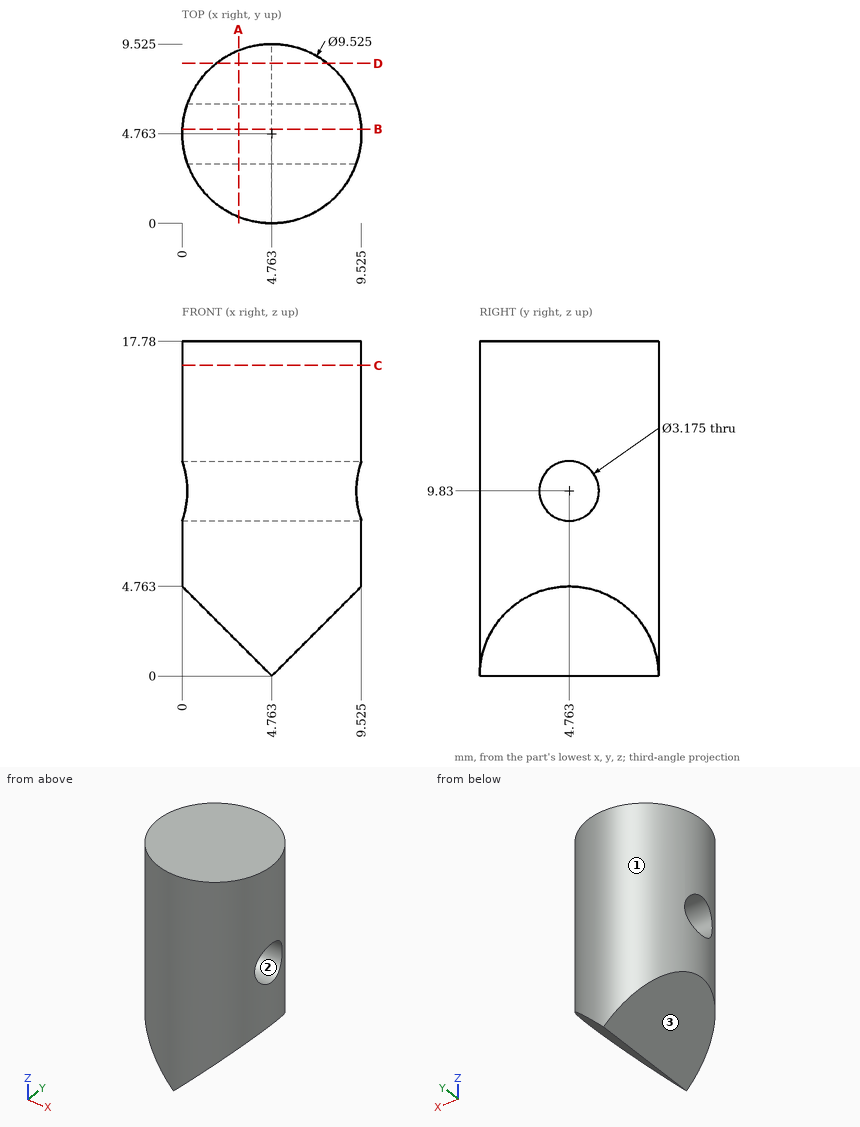
The drawing under review shows one solid part. Ordinate dimensions are in mm from its lowest x, y, z. Round coordinates to 2 decimals unless told otherwise and drop trailing zeros. Write each loop counter-clockwise with the first axis right and the second up, starting at its lowest first coordinate (ties: lowest second). Pieces come first, ordered by that corner, then holes.
(1) Mouldability with a two-part tool opening along Z and no side actions: class the marked faces 1, 2 and 3 as +Z half, -Z half, draft (parallel to the pull), parting line (faces both ways), or undercut.
(2) We need section C-C on z = 16.5. Give the boundary of the cut face in (x, y) (1 decimal).
(3) Insertion check: pin 1 (3 mm diameter, centred on y = 2, z = 3.5, fed in from +X); pin 2 (4 mm diameter, centred on y = 8, z = 5.5, fed in from +X); pin 3 (4 mm diameter, centred on y = 7, z = 7.5, fed in from +X). Each pin has a flat end and moves straight along its axis. Give the tip position at first contact, or say it passes through.
(4) We need section B-B on y = 5. Give the boundary of the cut face in (x, z) (1 decimal).
(5) We need section A-A on x = 3. Give the boundary of the cut face in (y, z) (1 decimal).
(6) Wall thickness on L1, parallel to Y at x = 5.25, z = 8.5 (1 decimal); L2, parallel to Y at x = 2, z = 8.5 (1 decimal); L3, parallel to Z at x = 3.25, y = 5.25 (1 decimal): over which ranges is each line inside the solid? List them lowest first.
(7) We need section D-D on y = 8.5. Give the boundary of the cut face in (x, z) (1 decimal).
Findings below:
1. face 1: draft
1. face 2: undercut
1. face 3: -Z half
2. outline: circle Ø9.5 at (4.8, 4.8)
3. pin 1: stops at x = 9.24
3. pin 2: stops at x = 9.36
3. pin 3: stops at x = 9.52
4. outline: (0, 4.8) - (4.8, 0) - (9.5, 4.8) - (9.5, 8.3) - (0, 8.3) - close; (0, 11.4) - (9.5, 11.4) - (9.5, 17.8) - (0, 17.8) - close
5. outline: (0.3, 1.8) - (9.2, 1.8) - (9.2, 17.8) - (0.3, 17.8) - close; hole circle Ø3.2 at (4.8, 9.8)
6. L1: y = 0 to 3.9, 5.6 to 9.5
6. L2: y = 0.9 to 3.9, 5.6 to 8.6
6. L3: z = 1.5 to 8.3, 11.3 to 17.8
7. outline: (1.8, 3) - (4.8, 0) - (7.7, 3) - (7.7, 17.8) - (1.8, 17.8) - close
